Geometry: final body of the model. Coordinates: model frame, mm. A direction names the side the tool comes from. Give positions to 0.01 mm unless a question says otherwise; leave off trailing zeros. Loops run counter-clockwise (first coordinate to the right, second up) from the corner with the lowest first, then second, coordinate; pieces in that order, holes last. Notation, with made-up numbers: (46.25, 27) - (70.25, 27) arc R12 cw to (70.25, 34) - close; hole circle Ø3 at (-18.5, 24). An arc over 180 degrees is marked (long way). Use one line per item in the form item = value.
```python
from build123d import *
from OCP.BRepFilletAPI import BRepFilletAPI_MakeChamfer

# Parameters (mm, degrees)
SKETCH1_W           = 11.64
SKETCH1_H           = 23.7
BOSS_EXTRUDE1_DEPTH = 20.25
SKETCH2_W           = 11.64
SKETCH2_H           = 2
BOSS_EXTRUDE2_DEPTH = 4.45
SKETCH3_W           = 11.64
SKETCH3_H           = 2
BOSS_EXTRUDE3_DEPTH = 4.45
FILLET1_R           = 1
BOSS_EXTRUDE4_DEPTH = 6
CHAMFER2_SIZE2      = 1.400415076
CHAMFER2_SIZE       = 2
SKETCH5_R           = 2.5
BOSS_EXTRUDE5_DEPTH = 3.25
SKETCH6_W           = 6
SKETCH6_H           = 4
SKETCH6_W_2         = 3.2
SKETCH6_H_2         = 1.2
BOSS_EXTRUDE6_DEPTH = 1.5
FILLET2_R           = 0.5
CHAMFER3_SIZE       = 0.5
CHAMFER3_SIZE2      = 0.350103769
CUT_EXTRUDE1_REACH  = 27.887
SKETCH7_R           = 1.016
FILLET3_R           = 0.5


with BuildPart() as part:
    # Sketch1 → Boss-Extrude1 (new body)
    with BuildSketch(Plane(origin=(0, 0, 0), x_dir=(1, 0, 0), z_dir=(0, 1, 0))):
        Rectangle(SKETCH1_W, SKETCH1_H)
    extrude(amount=BOSS_EXTRUDE1_DEPTH)

    # Sketch2 → Boss-Extrude2 (add)
    with BuildSketch(Plane.XY.offset(11.85)):
        with Locations((0, 18.25)):
            Rectangle(SKETCH2_W, SKETCH2_H)
    extrude(amount=BOSS_EXTRUDE2_DEPTH)

    # Sketch3 → Boss-Extrude3 (add)
    with BuildSketch(Plane(origin=(0, 0, -11.85), x_dir=(-1, 0, 0), z_dir=(0, 0, -1))):
        with Locations((0, 18.25)):
            Rectangle(SKETCH3_W, SKETCH3_H)
    extrude(amount=BOSS_EXTRUDE3_DEPTH)

    # Fillet1
    fillet1_edges = [part.edges().sort_by_distance(p)[0] for p in [
        (5.82, 8.625, 11.85),
        (-5.82, 8.625, 11.85),
        (5.82, 18.25, 16.3),
        (-5.82, 18.25, 16.3),
        (-5.82, 8.625, -11.85),
        (5.82, 8.625, -11.85),
        (-5.82, 18.25, -16.3),
        (5.82, 18.25, -16.3),
        (5.82, 19.75, 11.85),
        (-5.82, 19.75, 11.85),
        (-5.82, 19.75, -11.85),
        (5.82, 19.75, -11.85),
    ]]
    fillet(fillet1_edges, radius=FILLET1_R)

    # Sketch4 → Boss-Extrude4 (add)
    with BuildSketch(Plane(origin=(0, 20.25, 0), x_dir=(1, 0, 0), z_dir=(0, 1, 0))):
        with BuildLine():
            Line((-3, -0.15), (-3, 0.611197026))
            ThreePointArc((-3, 0.611197026), (-4.778645953, 2.169252733), (-5.82, 4.292151873))
            Line((-5.82, 4.292151873), (-5.82, 7.368248127))
            ThreePointArc((-5.82, 7.368248127), (0, 11.85), (5.82, 7.368248127))
            Line((5.82, 7.368248127), (5.82, 4.292151873))
            ThreePointArc((5.82, 4.292151873), (4.778645953, 2.169252733), (3, 0.611197026))
            Line((3, 0.611197026), (3, -0.15))
            ThreePointArc((3, -0.15), (0, -3.15), (-3, -0.15))
        make_face()
    extrude(amount=BOSS_EXTRUDE4_DEPTH)

    # Chamfer2
    chamfer2_edges = [part.edges().sort_by_distance(p)[0] for p in [
        (-5.82, 26.25, -5.8302),
    ]]
    chamfer2_side = [part.faces().sort_by_distance(p)[0] for p in [
        (-5.82, 26.221991698, -5.8302),
    ]]
    chamfer(chamfer2_edges, length=CHAMFER2_SIZE, length2=CHAMFER2_SIZE2, reference=chamfer2_side[0])
    chamfer2_2_edges = [part.edges().sort_by_distance(p)[0] for p in [
        (5.82, 26.25, -5.8302),
    ]]
    chamfer2_2_side = [part.faces().sort_by_distance(p)[0] for p in [
        (5.791991698, 26.25, -5.8302),
    ]]
    chamfer(chamfer2_2_edges, length=CHAMFER2_SIZE2, length2=CHAMFER2_SIZE, reference=chamfer2_2_side[0])
    chamfer2_3_edges = [part.edges().sort_by_distance(p)[0] for p in [
        (3.752705775, 26.25, -1.123269853),
    ]]
    chamfer2_3_side = [part.faces().sort_by_distance(p)[0] for p in [
        (3.735245575, 26.25, -1.14516977),
    ]]
    chamfer(chamfer2_3_edges, length=CHAMFER2_SIZE2, length2=CHAMFER2_SIZE, reference=chamfer2_3_side[0])
    chamfer2_4_edges = [part.edges().sort_by_distance(p)[0] for p in [
        (-3.752705775, 26.25, -1.123269853),
    ]]
    chamfer2_4_side = [part.faces().sort_by_distance(p)[0] for p in [
        (-3.735245575, 26.25, -1.14516977),
    ]]
    chamfer(chamfer2_4_edges, length=CHAMFER2_SIZE2, length2=CHAMFER2_SIZE, reference=chamfer2_4_side[0])
    chamfer2_5_edges_1 = [part.edges().sort_by_distance(p)[0] for p in [
        (3, 26.25, -0.230598513),
    ]]
    chamfer2_5_side_1 = [part.faces().sort_by_distance(p)[0] for p in [
        (2.971991698, 26.25, -0.230598513),
    ]]
    chamfer2_5_edges_2 = [part.edges().sort_by_distance(p)[0] for p in [
        (0, 26.25, 3.15),
    ]]
    chamfer2_5_side_2 = [part.faces().sort_by_distance(p)[0] for p in [
        (0, 26.25, 3.121991698),
    ]]
    chamfer2_5_edges_3 = [part.edges().sort_by_distance(p)[0] for p in [
        (-3, 26.25, -0.230598513),
    ]]
    chamfer2_5_side_3 = [part.faces().sort_by_distance(p)[0] for p in [
        (-2.971991698, 26.25, -0.230598513),
    ]]
    chamfer2_5 = BRepFilletAPI_MakeChamfer(part.part.solid().wrapped)
    for e in chamfer2_5_edges_1:
        chamfer2_5.Add(CHAMFER2_SIZE2, CHAMFER2_SIZE, e.wrapped, chamfer2_5_side_1[0].wrapped)
    for e in chamfer2_5_edges_2:
        chamfer2_5.Add(CHAMFER2_SIZE2, CHAMFER2_SIZE, e.wrapped, chamfer2_5_side_2[0].wrapped)
    for e in chamfer2_5_edges_3:
        chamfer2_5.Add(CHAMFER2_SIZE2, CHAMFER2_SIZE, e.wrapped, chamfer2_5_side_3[0].wrapped)
    add(Compound.cast(chamfer2_5.Shape()), mode=Mode.REPLACE)
    chamfer2_6_edges = [part.edges().sort_by_distance(p)[0] for p in [
        (0, 26.25, -11.85),
    ]]
    chamfer2_6_side = [part.faces().sort_by_distance(p)[0] for p in [
        (0, 26.25, -11.821991698),
    ]]
    chamfer(chamfer2_6_edges, length=CHAMFER2_SIZE2, length2=CHAMFER2_SIZE, reference=chamfer2_6_side[0])

    # Sketch5 → Boss-Extrude5 (add)
    with BuildSketch(Plane(origin=(0, 26.25, 0), x_dir=(1, 0, 0), z_dir=(0, 1, 0))):
        with Locations(Location((0, 5.8302, 0), (0, 0, 90))):
            Circle(SKETCH5_R)
    extrude(amount=BOSS_EXTRUDE5_DEPTH)

    # Sketch6 → Boss-Extrude6 (add)
    with BuildSketch(Plane(origin=(0, 0, -11.85), x_dir=(-1, 0, 0), z_dir=(0, 0, -1))):
        with Locations((0, 3)):
            Rectangle(SKETCH6_W, SKETCH6_H)
        with Locations((0, 3)):
            Rectangle(SKETCH6_W_2, SKETCH6_H_2, mode=Mode.SUBTRACT)
    extrude(amount=BOSS_EXTRUDE6_DEPTH)

    # Fillet2
    fillet2_edges = [part.edges().sort_by_distance(p)[0] for p in [
        (-3, 1, -12.6),
        (-3, 5, -12.6),
        (3, 5, -12.6),
        (3, 1, -12.6),
        (1.6, 3.6, -12.6),
        (1.6, 2.4, -12.6),
        (-1.6, 2.4, -12.6),
        (-1.6, 3.6, -12.6),
    ]]
    fillet(fillet2_edges, radius=FILLET2_R)

    # Chamfer3
    chamfer3_edges = [part.edges().sort_by_distance(p)[0] for p in [
        (0, 29.5, -3.3302),
    ]]
    chamfer3_side = [part.faces().sort_by_distance(p)[0] for p in [
        (0, 27.875, -3.3302),
    ]]
    chamfer(chamfer3_edges, length=CHAMFER3_SIZE, length2=CHAMFER3_SIZE2, reference=chamfer3_side[0])

    # Sketch7 → Cut-Extrude1 (cut, up to next)
    with BuildSketch(Plane(origin=(0, 19.25, 0), x_dir=(1, 0, 0), z_dir=(0, 1, 0)), mode=Mode.PRIVATE) as cut_extrude1_sk1:
        with Locations(Location((0, -14.1605, 0), (0, 0, 270))):
            Circle(SKETCH7_R)
    cut_extrude1_tool1 = extrude(cut_extrude1_sk1.sketch, amount=-CUT_EXTRUDE1_REACH, mode=Mode.PRIVATE) & part.part
    # Sketch7 → Cut-Extrude1 (cut, up to next)
    with BuildSketch(Plane(origin=(0, 19.25, 0), x_dir=(1, 0, 0), z_dir=(0, 1, 0)), mode=Mode.PRIVATE) as cut_extrude1_sk2:
        with Locations(Location((0, 14.1605, 0), (0, 0, 270))):
            Circle(SKETCH7_R)
    cut_extrude1_tool2 = extrude(cut_extrude1_sk2.sketch, amount=-CUT_EXTRUDE1_REACH, mode=Mode.PRIVATE) & part.part
    # Sketch7 → Cut-Extrude1 (cut, up to next)
    with BuildSketch(Plane(origin=(0, 19.25, 0), x_dir=(1, 0, 0), z_dir=(0, 1, 0)), mode=Mode.PRIVATE) as cut_extrude1_sk3:
        with Locations(Location((-3.302, 13.6525, 0), (0, 0, 270))):
            Circle(SKETCH7_R)
    cut_extrude1_tool3 = extrude(cut_extrude1_sk3.sketch, amount=-CUT_EXTRUDE1_REACH, mode=Mode.PRIVATE) & part.part
    # Sketch7 → Cut-Extrude1 (cut, up to next)
    with BuildSketch(Plane(origin=(0, 19.25, 0), x_dir=(1, 0, 0), z_dir=(0, 1, 0)), mode=Mode.PRIVATE) as cut_extrude1_sk4:
        with Locations(Location((3.302, 13.6525, 0), (0, 0, 270))):
            Circle(SKETCH7_R)
    cut_extrude1_tool4 = extrude(cut_extrude1_sk4.sketch, amount=-CUT_EXTRUDE1_REACH, mode=Mode.PRIVATE) & part.part
    # Sketch7 → Cut-Extrude1 (cut, up to next)
    with BuildSketch(Plane(origin=(0, 19.25, 0), x_dir=(1, 0, 0), z_dir=(0, 1, 0)), mode=Mode.PRIVATE) as cut_extrude1_sk5:
        with Locations(Location((-3.302, -13.6525, 0), (0, 0, 270))):
            Circle(SKETCH7_R)
    cut_extrude1_tool5 = extrude(cut_extrude1_sk5.sketch, amount=-CUT_EXTRUDE1_REACH, mode=Mode.PRIVATE) & part.part
    # Sketch7 → Cut-Extrude1 (cut, up to next)
    with BuildSketch(Plane(origin=(0, 19.25, 0), x_dir=(1, 0, 0), z_dir=(0, 1, 0)), mode=Mode.PRIVATE) as cut_extrude1_sk6:
        with Locations(Location((3.302, -13.6525, 0), (0, 0, 270))):
            Circle(SKETCH7_R)
    cut_extrude1_tool6 = extrude(cut_extrude1_sk6.sketch, amount=-CUT_EXTRUDE1_REACH, mode=Mode.PRIVATE) & part.part
    add(cut_extrude1_tool1.solids().sort_by_distance((0, 19.25, 14.1605))[0], mode=Mode.SUBTRACT)
    add(cut_extrude1_tool2.solids().sort_by_distance((0, 19.25, -14.1605))[0], mode=Mode.SUBTRACT)
    add(cut_extrude1_tool3.solids().sort_by_distance((-3.302, 19.25, -13.6525))[0], mode=Mode.SUBTRACT)
    add(cut_extrude1_tool4.solids().sort_by_distance((3.302, 19.25, -13.6525))[0], mode=Mode.SUBTRACT)
    add(cut_extrude1_tool5.solids().sort_by_distance((-3.302, 19.25, 13.6525))[0], mode=Mode.SUBTRACT)
    add(cut_extrude1_tool6.solids().sort_by_distance((3.302, 19.25, 13.6525))[0], mode=Mode.SUBTRACT)

    # Fillet3
    fillet3_edges = [part.edges().sort_by_distance(p)[0] for p in [
        (0, 1, -13.35),
        (3, 3, -13.35),
        (-3, 3, -13.35),
        (0, 5, -13.35),
        (2.853553391, 4.853553391, -13.35),
        (-2.853553391, 4.853553391, -13.35),
        (-2.853553391, 1.146446609, -13.35),
        (2.853553391, 1.146446609, -13.35),
    ]]
    fillet(fillet3_edges, radius=FILLET3_R)


solid = part.part
```
(1) Material intervals for L1, parallel to Y at x = 3, z = 5; L2, parallel to Z at x = -2, y = 14.25; L3, parallel to Y at x = -3, z = -9, sorted ascending. Write a range as from..to.
Solution:
L1 = 0..20.25
L2 = -11.85..11.85
L3 = 0..26.25
(2) Cut plane A-A (y = 10.5). Return the cut outline in (x, z).
Solution:
outline = (-5.82, -10.85) arc R1 ccw to (-4.82, -11.85) - (4.82, -11.85) arc R1 ccw to (5.82, -10.85) - (5.82, 10.85) arc R1 ccw to (4.82, 11.85) - (-4.82, 11.85) arc R1 ccw to (-5.82, 10.85) - close
(3) Pull-direction query (Z, two-part tool) for faces 6 (the face through (-4.758, 22.222, -2.143)), 7 (the face through (-2.997, 18.264, 14.622)), 8 (the face through (0, 5, -12)); classes: released by +Z, released by -Z, zero draft, split by the parting line, or undercut.
Solution:
face_6 = released by +Z
face_7 = undercut
face_8 = zero draft
(4) Access query for faces 1 (the face through (-4, 20.25, -11)), 2 (the face through (-5.535, 8.746, 11.549)), 3 (the face through (-5.535, 19.757, 11.549)), 4 (the face through (5.519, 8.746, 11.565)), 5 (the face through (0.305, 18.264, -13.191)). Directions: +Z, -Z, +X, -X, +Y, -Y. A direction counts if a zero-diameter tool reaches every point of the face in a straight line with its end or side. Return the directions, or none.
Solution:
face_1 = -Z, -X, +Y
face_2 = +Z, -X, -Y
face_3 = +Z, -X, +Y
face_4 = +Z, +X, -Y
face_5 = +Y
(5) Cut plane B-B (z = 6). Return the cut outline in (x, y).
Solution:
outline = (-5.82, 0) - (5.82, 0) - (5.82, 20.25) - (-5.82, 20.25) - close
(6) Pin query (flat end, axial travel): P1, Ø0.5, axis at y = 2.5, z = -12.5, coming from the +X side; P2, Ø6, axis at x = 2.5, z = 14.5, coming from the -Y side; P3, Ø3.5, axis at x = -4, z = -10.5, coming from the +Y side; P4, Ø5, axis at x = 1.5, y = 8.5, coming from the +Z side. Return the tip coordinate at first contact, or that it passes through.
Solution:
P1 = 3
P2 = 0
P3 = 26.25
P4 = 11.85
(7) Cut plane C-C (y = 23.5). Return the cut outline in (x, z).
Solution:
outline = (-5.82, -7.37) arc R6.02 ccw to (5.82, -7.37) - (5.82, -4.29) arc R6.02 ccw to (3, -0.61) - (3, 0.15) arc R3 ccw to (-3, 0.15) - (-3, -0.61) arc R6.02 ccw to (-5.82, -4.29) - close
